CAD build for the part. Positions are in the model's coordinates, mm. Round coordinates to 2 decimals unless told otherwise and drop trailing zeros. Order: outer loops, then holes, each group sorted by start corner. A loop starts at its lowest first (then second) coordinate and runs counter-clockwise, first axis right, second up. Notation, with made-up numbers: M -28.5,-37 L 22.5,-37 A15 cw 22.5,-8 Z; hole C 62,33 d5. An arc over 180 degrees is marked long. Put each result on its own line as item: value.
```python
from build123d import *

# Parameters (mm, degrees)
F0_R     = 5
F1_DEPTH = 5


with BuildPart() as f1:
    # F0 (on Front) → F1 (new body)
    with BuildSketch(Plane.XZ):
        with BuildLine():
            ThreePointArc((0, 25), (-12.5, 12.5), (0, 0))
            Line((0, 0), (200, 0))
            ThreePointArc((200, 0), (212.5, 12.5), (200, 25))
            Line((200, 25), (0, 25))
        make_face()
        with BuildLine():
            ThreePointArc((0, 7.5), (-5, 12.5), (0, 17.5))
            ThreePointArc((0, 17.5), (3.535534, 16.035534), (5, 12.5))
            ThreePointArc((5, 12.5), (3.535534, 8.964466), (0, 7.5))
        make_face(mode=Mode.SUBTRACT)
        with BuildLine():
            ThreePointArc((80, 12.5), (78.535534, 8.964466), (75, 7.5))
            ThreePointArc((75, 7.5), (70, 12.5), (75, 17.5))
            ThreePointArc((75, 17.5), (78.535534, 16.035534), (80, 12.5))
        make_face(mode=Mode.SUBTRACT)
        with Locations((200, 12.5)):
            Circle(F0_R, mode=Mode.SUBTRACT)
    extrude(amount=F1_DEPTH)


solid = f1.part
```
Item 1: Pin check, flat tips, straight feed: P1, Ø1.5, axis at y = -1.5, z = 11, coming from the -X side; P2, Ø1.5, axis at y = -2, z = 18.5, coming from the +X side. Stop position of each tip, or through.
Answers below:
P1: x = -12.48
P2: x = 211.34
Item 2: Band-saw the part on A-A on y = -2.9. Give the cut face in (x, z).
Answers below:
outline: M 0,0 L 200,0 A12.5 ccw 200,25 L 0,25 A12.5 ccw Z; hole C 0,12.5 d10; hole C 75,12.5 d10; hole C 200,12.5 d10
Item 3: Probe line 1 along Z through (x, y) = (200, -2.4); line 2 along X through (y, z) = (-0.95, 13); line 3 along X through (y, z) = (-0.9, 9.5). List the from-to ranges inside material, lowest first. Write a range as [from, to].
Answers below:
line 1: [0, 7.5], [17.5, 25]
line 2: [-12.49, -4.97], [4.97, 70.03], [79.97, 195.03], [204.97, 212.49]
line 3: [-12.13, -4], [4, 71], [79, 196], [204, 212.13]
Item 4: Band-saw the part on B-B on z = 21. Give the cut face in (x, y).
Answers below:
outline: M -9.17,-5 L 209.17,-5 L 209.17,0 L -9.17,0 Z
Item 5: Mould opens along X. For faces 1 (the flat face through (99, -2, 0)), 2 (the cylindrical face through (212.497, -2.465, 12.225)), 3 (the cylindrical face through (204.77, -2.46, 14)), 4 (the cylindrical face through (-12.497, -2.465, 12.775)) say: pulls with the +X half, pulls with the -X half, needs draft (parallel to the pull), parting line crosses it, or undercut.
Answers below:
face 1: needs draft
face 2: pulls with the +X half
face 3: undercut
face 4: pulls with the -X half
